```python
from build123d import *

# Parameters (mm, degrees)
F1_DEPTH      = 1.016
F1_DEPTH_BACK = 1.016
F2_DEPTH      = 0.7112
F2_DEPTH_BACK = 0.7112
F4_DEPTH      = 25.4


with BuildPart() as f1:
    # F0 (on Front) → F1 (new body, two sides)
    with BuildSketch(Plane.XZ) as f1_sk:
        with BuildLine():
            Line((-4.6784887666, 4.3793842609), (1.5288887666, 4.3793842609))
            Line((1.5288887666, 4.3793842609), (3.7084, 4.3793842609))
            Line((3.7084, 4.3793842609), (3.7084, 5.2683842609))
            Line((3.7084, 5.2683842609), (-1.5748, 6.985))
            ThreePointArc((-1.5748, 6.985), (-4.3539247834, 6.5499498923), (-6.858, 5.2683842609))
            Line((-6.858, 5.2683842609), (-6.858, 4.3793842609))
            Line((-6.858, 4.3793842609), (-4.6784887666, 4.3793842609))
        make_face()
    extrude(amount=F1_DEPTH)
    extrude(f1_sk.sketch, amount=-F1_DEPTH_BACK)

    # F0 (on Front) → F2 (join, two sides)
    with BuildSketch(Plane.XZ) as f2_sk:
        with BuildLine():
            Line((-3.1496, 0), (0, 0))
            Line((0, 0), (0, 3.1198752576))
            ThreePointArc((0, 3.1198752576), (0.8477307051, 3.6485304249), (1.5288887666, 4.3793842609))
            Line((1.5288887666, 4.3793842609), (-4.6784887666, 4.3793842609))
            ThreePointArc((-4.6784887666, 4.3793842609), (-3.9973307051, 3.6485304249), (-3.1496, 3.1198752576))
            Line((-3.1496, 3.1198752576), (-3.1496, 0))
        make_face()
    extrude(amount=F2_DEPTH)
    extrude(f2_sk.sketch, amount=-F2_DEPTH_BACK)

    # F3 (on face) → F4 (cut)
    with BuildSketch(Plane.XZ.offset(1.016)):
        Polygon((-1.2099161613, 6.65278493), (-0.9538692542, 6.7832473707), (-1.3403786224, 6.9088318772), align=None)
        Polygon((-0.8234067931, 6.5272004235), (-0.567359886, 6.6576628642), (-0.9538692542, 6.7832473707), align=None)
        Polygon((-0.4368974248, 6.401615917), (-0.1808505177, 6.5320783577), (-0.567359886, 6.6576628642), align=None)
        Polygon((-0.0503880566, 6.2760314105), (0.2056588505, 6.4064938511), (-0.1808505177, 6.5320783577), align=None)
        Polygon((0.3361213116, 6.1504469039), (0.5921682187, 6.2809093446), (0.2056588505, 6.4064938511), align=None)
        Polygon((0.7226306798, 6.0248623974), (0.9786775869, 6.1553248381), (0.5921682187, 6.2809093446), align=None)
        Polygon((1.1091400481, 5.8992778909), (1.3651869552, 6.0297403316), (0.9786775869, 6.1553248381), align=None)
        Polygon((1.4956494163, 5.7736933844), (1.7516963234, 5.9041558251), (1.3651869552, 6.0297403316), align=None)
        Polygon((1.8821587845, 5.6481088779), (2.1382056916, 5.7785713186), (1.7516963234, 5.9041558251), align=None)
        Polygon((2.2686681527, 5.5225243714), (2.5247150598, 5.6529868121), (2.1382056916, 5.7785713186), align=None)
        Polygon((2.6551775209, 5.3969398649), (2.911224428, 5.5274023055), (2.5247150598, 5.6529868121), align=None)
        Polygon((3.0416868892, 5.2713553583), (3.2977337963, 5.401817799), (2.911224428, 5.5274023055), align=None)
    extrude(amount=-F4_DEPTH, mode=Mode.SUBTRACT)


solid = f1.part
```
Here's how the part is built. I have some questions about the finished solid (model axes, mm). A direction names the side the tool comes from. Give positions to 0.01 mm unless a question says otherwise; leave off trailing zeros. Order: outer loops, then holes, each group sorted by start corner. A loop starts at its lowest first (then second) coordinate and runs counter-clockwise, first axis right, second up. Notation, with made-up numbers: (35, 1) - (55, 1) arc R10 cw to (55, 19) - close; hole circle Ø11 at (-7, -7). An arc over 180 degrees is marked (long way). Answer as a JSON object with one key per item and string values. Group by question number.
Item 1: If we section it at B-B on z = 2: Please give me the cut outline in (x, y), and give its area (3 significant figures).
Item 2: If we section it at D-D on x = -4.5: Please give me the cut outline in (y, z), and give its area (3 significant figures).
Item 3: For P1, Ø0.7, axis at y = 0, z = 1, coming from the -X side; P2, Ø2, axis at x = -0.5, z = 2.5, coming from the +Y side; P3, Ø1.3, axis at x = -1, z = 2, coming from the -Y side, each with a flat end and sliding along its axis, tell me the tip position at first contact or that it passes through.
Item 4: Please list where these lines run through material, in increasing order: probe 1 along Y at (x, z) = (-2.5, 3.25); probe 2 along X at (y, z) = (-0.1, 2); probe 3 along Z at (x, y) = (-2.75, 0.4).
Item 5: Which directions (+Z, -Z, +X, -X, +Y, -Y) give clear straight access to the entire face, cutting with the end or side of a thin tool? Please do faces 1 (the flat face through (0, 0, 2)), 2 (the flat face through (-2, -0.711, 2)), 3 (the flat face through (-2, 0.711, 2)).
Item 6: If we section it at C-C on x = -3: Please give me the cut outline in (y, z), and give its area (3 significant figures).
Result set:
{
 "1": {"outline": "(-3.15, -0.71) - (0, -0.71) - (0, 0.71) - (-3.15, 0.71) - close", "area": "4.48 mm²"},
 "2": {"outline": "(-1.02, 4.38) - (-0.71, 4.38) - (-0.71, 4.15) - (0.71, 4.15) - (0.71, 4.38) - (1.02, 4.38) - (1.02, 6.5) - (-1.02, 6.5) - close", "area": "4.64 mm²"},
 "3": {"P1": "x = -3.15", "P2": "y = 0.71", "P3": "y = -0.71"},
 "4": {"probe 1": "-0.71 to 0.71", "probe 2": "-3.15 to 0", "probe 3": "0 to 6.91"},
 "5": {"face 1": "-Z, +X, +Y, -Y", "face 2": "-Z, +X, -X, -Y", "face 3": "-Z, +X, -X, +Y"},
 "6": {"outline": "(-1.02, 4.38) - (-0.71, 4.38) - (-0.71, 0) - (0.71, 0) - (0.71, 4.38) - (1.02, 4.38) - (1.02, 6.88) - (-1.02, 6.88) - close", "area": "11.3 mm²"}
}
